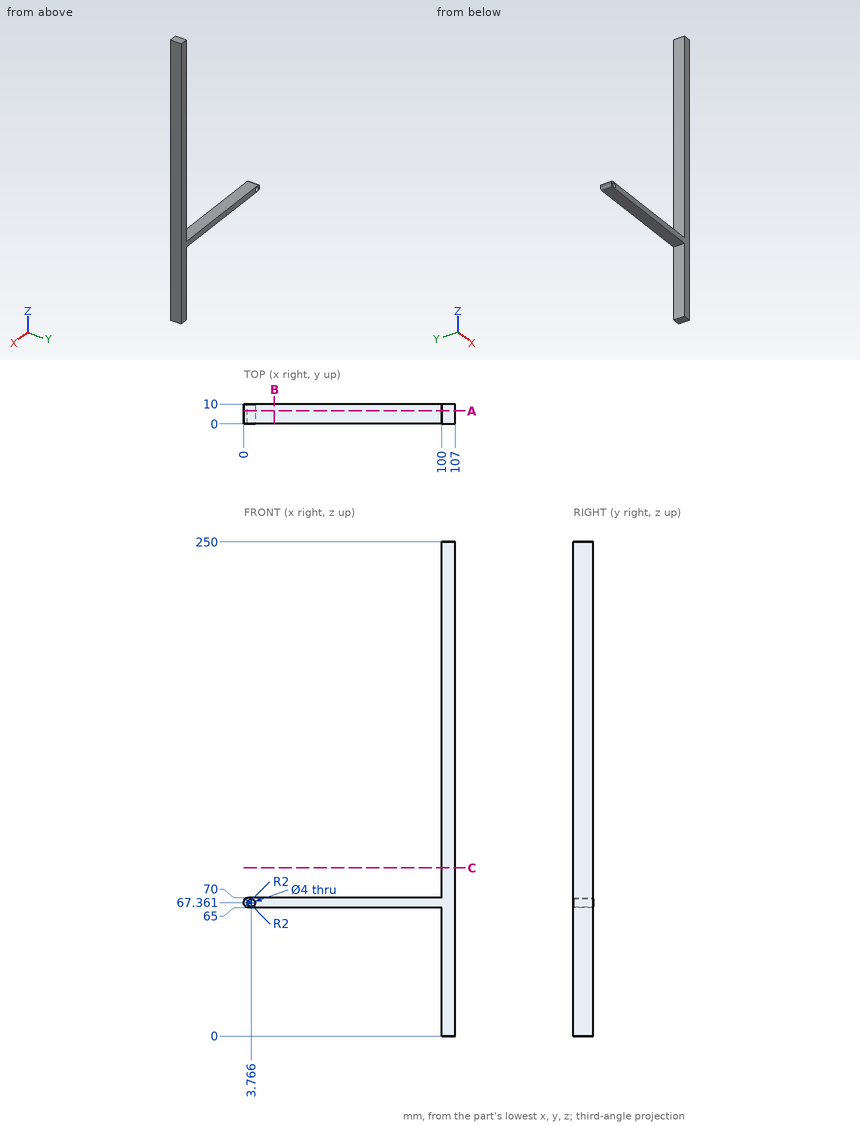
Here's the drawing with two shaded views (mm, measured from the low corner). I have some questions. Give positions to 0.01 mm unless a question says otherwise; leave off trailing zeros. Order: outer loops, then holes, each group sorted by start corner. A loop starts at its lowest first (then second) coordinate and runs counter-clockwise, first axis right, second up. Notation, with made-up numbers: M 4,17 L 26,17 A25 ccw 26,43 Z; hole C -39,40 d11. An arc over 180 degrees is marked long. One line per item, written item: value.
1) I want a section at A-A, the plane y = 6.5. List the corners of the cut face in (x, z) for me.
Answer sheet:
outline: M 0,67 A2 ccw 2,65 L 100,65 L 100,0 L 107,0 L 107,250 L 100,250 L 100,70 L 2,70 A2 ccw 0,68 Z; hole C 3.77,67.36 d4
2) For P1, Ø5, axis at y = 7.5, z = 42.5, coming from the -X side; P2, Ø4, axis at x = 31.5, y = 4, coming from the -Z side; P3, Ø4, axis at x = 73.5, y = 1.5, coming from the +Z side, each with a flat end and sliding along its axis, tell me the tip position at first contact or that it passes through.
Answer sheet:
P1: stops at x = 100
P2: stops at z = 65
P3: stops at z = 70
3) I want a section at C-C, the plane z = 85. List the corners of the cut face in (x, y) for me.
Answer sheet:
outline: M 100,0 L 107,0 L 107,10 L 100,10 Z
4) Please list where these lines run through material, in increasing order: line 1 along Z through (x, y) = (8.5, 2); line 2 along X through (y, z) = (3.5, 39.5).
Answer sheet:
line 1: z = 65 to 70
line 2: x = 100 to 107
5) I want a section at B-B, the plane x = 15.5. List the corners of the cut face in (y, z) for me, plus the area to 3 significant figures.
Answer sheet:
outline: M 0,65 L 10,65 L 10,70 L 0,70 Z
area: 50.0 mm^2
